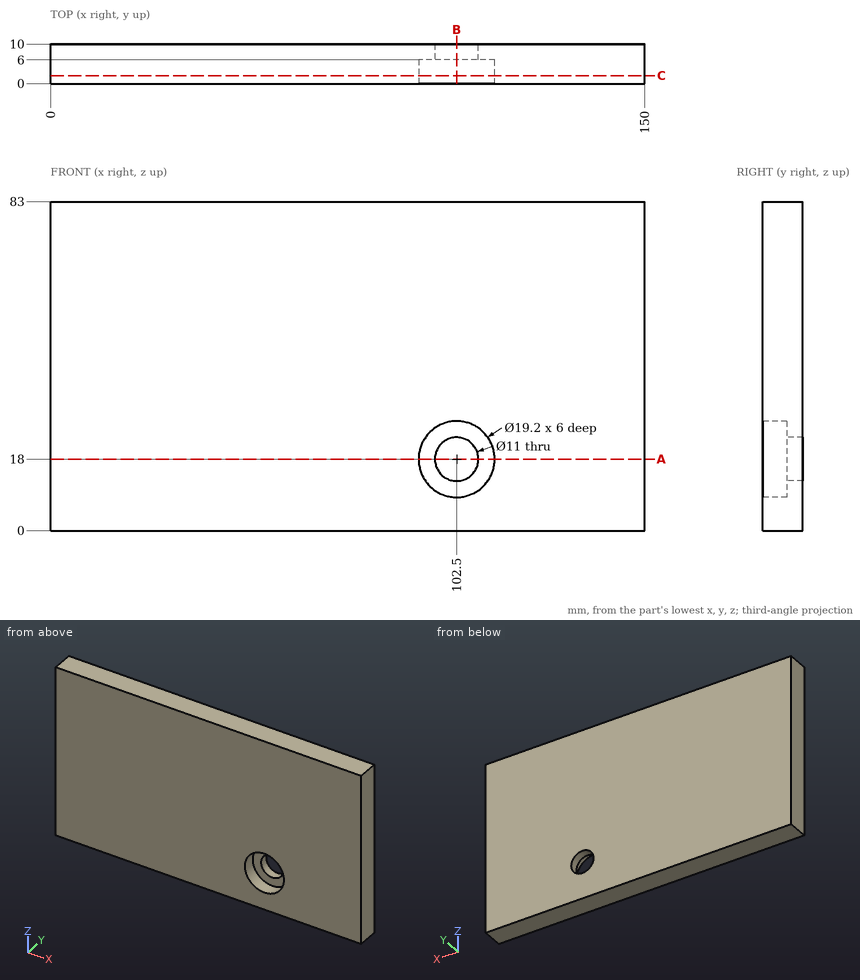
Input: dimensioned drawing with shaded views. Units: mm. Origin: part minimum x, y, z. Give positions to 0.01 mm unless a question says otherwise; leave off trailing zeros. Write each loop counter-clockwise with the first axis right and the second up, starting at its lowest first coordinate (ties: lowest second). Pieces come first, ordered by that corner, then holes. Notation, with made-up numbers: M 57.25,73.25 L 80.25,73.25 A35 ccw 80.25,109.25 Z; hole C 11.5,57.25 d2. An arc over 180 degrees is marked long. Return JSON: item names as keys, results as strings. Group by question number.
1) Cut plane B-B, the plane x = 102.5. Output: boundary loops of the cut face in (y, z).
2) Cut plane C-C, the plane y = 2. Output: boundary loops of the cut face in (x, z), plus the area to 3 significant figures.
3) Cut plane A-A, the plane z = 18. Output: boundary loops of the cut face in (x, y), plus the area to 3 significant figures.
4) Material intervals for line 1 along Z through (x, y) = (102.5, 6.8); line 2 along X through (y, z) = (3.25, 19); line 3 along Y through (x, z) = (109.5, 23.5), sorted ascending. Write a range as [from, to].
Recorded:
{
 "1": {"outline": "M 0,0 L 10,0 L 10,12.5 L 6,12.5 L 6,8.4 L 0,8.4 Z; M 0,27.6 L 6,27.6 L 6,23.5 L 10,23.5 L 10,83 L 0,83 Z"},
 "2": {"outline": "M 0,0 L 150,0 L 150,83 L 0,83 Z; hole C 102.5,18 d19.2", "area": "12,200 mm²"},
 "3": {"outline": "M 0,0 L 92.9,0 L 92.9,6 L 97,6 L 97,10 L 0,10 Z; M 108,6 L 112.1,6 L 112.1,0 L 150,0 L 150,10 L 108,10 Z", "area": "1,340 mm²"},
 "4": {"line 1": "z = [0, 12.5], [23.5, 83]", "line 2": "x = [0, 92.95], [112.05, 150]", "line 3": "y = [6, 10]"}
}
